The listing builds one solid part. Answer for the finished solid, in the listing's coordinates (mm). A direction names the side the tool comes from. Round coordinates to 2 decimals unless told otherwise and drop trailing zeros. Loops run counter-clockwise (first coordinate to the right, second up) from the corner with the lowest first, then second, coordinate; pieces in that order, holes last. Notation, with made-up numbers: (-3, 28) -> (16, 28) arc R29 ccw to (16, 59) -> close; hole circle Ø11 at (39.5, -14.5). An arc over 180 degrees is marked (long way). Use a Markdown table: item, result. Add a question column.
Q1. Section C-C on z = 8 is taken. Give the vertices of the cut face in (x, y).
Q2. Consider line 1 (X direction, y = 1.5, z = -14); line 2 (X direction, y = 1.25, z = 44); line 3 (X direction, y = 4.25, z = 44). Determine where each line is inside the solid, lowest interval first.
Q3. Section D-D on z = -10.5 is taken. Give the vertices of the cut face in (x, y), then the cut area to 3 significant figures.
Q4. Which of the six approach directions +Z, -Z, +X, -X, +Y, -Y give full straight-line access (tool end or side, diameter ignored) to faces 1 (the flat face through (-34, 9, 25)), 2 (the flat face through (-25.3, 5, -14)), 3 (the flat face through (39, 8, 1)), 4 (the flat face through (42.8, 3, -42.8))?
Q5. Section A-A on x = -44 is taken. Give the vertices of the cut face in (y, z), then the cut area to 3 significant figures.
Q6. Section B-B on z = -44 is taken. Give the vertices of the cut face in (x, y).
Q7. For a pull along X with two mould halves and no side action, classify faces 5 (the flat face through (8, 10, -9)), 6 (the flat face through (-16.4, 5, -14)), 7 (the flat face through (49, 2, 1)) as released by +X, released by -X, zero draft, split by the parting line, or undercut.
Q8. Given pin 1 Ø2 at (y, z) = (9, 27) entering from -X; pin 2 Ø6.5 at (x, z) = (44, 44) entering from +Y; pin 3 Ø1 at (x, z) = (-9, 13.5) entering from +Y, each flat-ended and moving along its own axis, determine where each tip first touches the part or whether it passes through.
from build123d import *

# Parameters (mm, degrees)
SKETCH1_W           = 98
SKETCH1_H           = 98
BOSS_EXTRUDE2_DEPTH = 10
SKETCH2_W           = 98
SKETCH2_H           = 98
SKETCH2_W_2         = 78
SKETCH2_H_2         = 78
CUT_EXTRUDE2_DEPTH  = 5
SKETCH3_R           = 2.75
CUT_EXTRUDE3_DEPTH  = 2
SKETCH4_R           = 1.5
CUT_EXTRUDE4_DEPTH  = 9
SKETCH6_W           = 50
SKETCH6_H           = 28
CUT_EXTRUDE6_DEPTH  = 2.5
CUT_EXTRUDE8_DEPTH  = 11.5


with BuildPart() as part:
    # Sketch1 → Boss-Extrude2 (new body)
    with BuildSketch(Plane(origin=(0, 0, 0), x_dir=(1, 0, 0), z_dir=(0, 1, 0))):
        Rectangle(SKETCH1_W, SKETCH1_H)
    extrude(amount=BOSS_EXTRUDE2_DEPTH)

    # Sketch2 → Cut-Extrude2 (cut)
    with BuildSketch(Plane(origin=(0, 10, 0), x_dir=(1, 0, 0), z_dir=(0, 1, 0))):
        Rectangle(SKETCH2_W, SKETCH2_H)
        Rectangle(SKETCH2_W_2, SKETCH2_H_2, mode=Mode.SUBTRACT)
    extrude(amount=-CUT_EXTRUDE2_DEPTH, mode=Mode.SUBTRACT)

    # Sketch3 → Cut-Extrude3 (cut)
    with BuildSketch(Plane(origin=(0, 5, 0), x_dir=(1, 0, 0), z_dir=(0, 1, 0))):
        with Locations(Location((-44, -44, 0), (0, 0, 270))):
            Circle(SKETCH3_R)
        with Locations(Location((44, -44, 0), (0, 0, 270))):
            Circle(SKETCH3_R)
        with Locations(Location((-44, 44, 0), (0, 0, 270))):
            Circle(SKETCH3_R)
        with Locations(Location((44, 44, 0), (0, 0, 270))):
            Circle(SKETCH3_R)
    extrude(amount=-CUT_EXTRUDE3_DEPTH, mode=Mode.SUBTRACT)

    # Sketch4 → Cut-Extrude4 (cut)
    with BuildSketch(Plane(origin=(0, 3, 0), x_dir=(1, 0, 0), z_dir=(0, 1, 0))):
        with Locations(Location((-44, 44, 0), (0, 0, 270))):
            Circle(SKETCH4_R)
        with Locations(Location((44, 44, 0), (0, 0, 270))):
            Circle(SKETCH4_R)
        with Locations(Location((44, -44, 0), (0, 0, 270))):
            Circle(SKETCH4_R)
        with Locations(Location((-44, -44, 0), (0, 0, 270))):
            Circle(SKETCH4_R)
    extrude(amount=-CUT_EXTRUDE4_DEPTH, mode=Mode.SUBTRACT)

    # Sketch6 → Cut-Extrude6 (cut)
    with BuildSketch(Plane(origin=(0, 10, 0), x_dir=(1, 0, 0), z_dir=(0, 1, 0))):
        with Locations((-9, -25)):
            Rectangle(SKETCH6_W, SKETCH6_H)
    extrude(amount=-CUT_EXTRUDE6_DEPTH, mode=Mode.SUBTRACT)

    # Sketch7 → Cut-Extrude8 (cut)
    with BuildSketch(Plane(origin=(0, 10, 0), x_dir=(1, 0, 0), z_dir=(0, 1, 0))):
        with BuildLine():
            ThreePointArc((-30.3, 32), (-29.714213562, 33.414213562), (-28.3, 34))
            Line((-28.3, 34), (-27.3, 34))
            ThreePointArc((-27.3, 34), (-25.885786438, 33.414213562), (-25.3, 32))
            Line((-25.3, 32), (-25.3, -4))
            ThreePointArc((-25.3, -4), (-25.885786438, -5.414213562), (-27.3, -6))
            Line((-27.3, -6), (-28.3, -6))
            ThreePointArc((-28.3, -6), (-29.714213562, -5.414213562), (-30.3, -4))
            Line((-30.3, -4), (-30.3, 32))
        make_face()
        with BuildLine():
            ThreePointArc((-14.4, -6), (-15.814213562, -5.414213562), (-16.4, -4))
            Line((-16.4, -4), (-16.4, 32))
            ThreePointArc((-16.4, 32), (-15.814213562, 33.414213562), (-14.4, 34))
            Line((-14.4, 34), (-13.4, 34))
            ThreePointArc((-13.4, 34), (-11.985786438, 33.414213562), (-11.4, 32))
            Line((-11.4, 32), (-11.4, -4))
            ThreePointArc((-11.4, -4), (-11.985786438, -5.414213562), (-13.4, -6))
            Line((-13.4, -6), (-14.4, -6))
        make_face()
        with BuildLine():
            ThreePointArc((-0.5, -6), (-1.914213562, -5.414213562), (-2.5, -4))
            Line((-2.5, -4), (-2.5, 32))
            ThreePointArc((-2.5, 32), (-1.914213562, 33.414213562), (-0.5, 34))
            Line((-0.5, 34), (0.5, 34))
            ThreePointArc((0.5, 34), (1.914213562, 33.414213562), (2.5, 32))
            Line((2.5, 32), (2.5, -4))
            ThreePointArc((2.5, -4), (1.914213562, -5.414213562), (0.5, -6))
            Line((0.5, -6), (-0.5, -6))
        make_face()
        with BuildLine():
            ThreePointArc((13.4, -6), (11.985786438, -5.414213562), (11.4, -4))
            Line((11.4, -4), (11.4, 32))
            ThreePointArc((11.4, 32), (11.985786438, 33.414213562), (13.4, 34))
            Line((13.4, 34), (14.4, 34))
            ThreePointArc((14.4, 34), (15.814213562, 33.414213562), (16.4, 32))
            Line((16.4, 32), (16.4, -4))
            ThreePointArc((16.4, -4), (15.814213562, -5.414213562), (14.4, -6))
            Line((14.4, -6), (13.4, -6))
        make_face()
        with BuildLine():
            ThreePointArc((27.3, -34), (25.885786438, -33.414213562), (25.3, -32))
            Line((25.3, -32), (25.3, -6))
            Line((25.3, -6), (25.3, 32))
            ThreePointArc((25.3, 32), (25.885786438, 33.414213562), (27.3, 34))
            Line((27.3, 34), (28.3, 34))
            ThreePointArc((28.3, 34), (29.714213562, 33.414213562), (30.3, 32))
            Line((30.3, 32), (30.3, -6))
            Line((30.3, -6), (30.3, -32))
            ThreePointArc((30.3, -32), (29.714213562, -33.414213562), (28.3, -34))
            Line((28.3, -34), (27.3, -34))
        make_face()
    extrude(amount=-CUT_EXTRUDE8_DEPTH, mode=Mode.SUBTRACT)


solid = part.part
Checked values:
| question | item | result |
|---|---|---|
| 1 | outline | (-49, 0) -> (25.3, 0) -> (25.3, 10) -> (-39, 10) -> (-39, 5) -> (-49, 5) -> close; (30.3, 0) -> (49, 0) -> (49, 5) -> (39, 5) -> (39, 10) -> (30.3, 10) -> close |
| 2 | line 1 | x = -49 to -30.3, -25.3 to -16.4, -11.4 to -2.5, 2.5 to 11.4, 16.4 to 25.3, 30.3 to 49 |
| 2 | line 2 | x = -49 to -45.5, -42.5 to 42.5, 45.5 to 49 |
| 2 | line 3 | x = -49 to -46.75, -41.25 to 41.25, 46.75 to 49 |
| 3 | outline | (-49, 0) -> (-30.3, 0) -> (-30.3, 10) -> (-39, 10) -> (-39, 5) -> (-49, 5) -> close; (-25.3, 0) -> (-16.4, 0) -> (-16.4, 10) -> (-25.3, 10) -> close; (-11.4, 0) -> (-2.5, 0) -> (-2.5, 10) -> (-11.4, 10) -> close; (2.5, 0) -> (11.4, 0) -> (11.4, 10) -> (2.5, 10) -> close; (16.4, 0) -> (25.3, 0) -> (25.3, 10) -> (16.4, 10) -> close; (30.3, 0) -> (49, 0) -> (49, 5) -> (39, 5) -> (39, 10) -> (30.3, 10) -> close |
| 3 | area | 630 mm2 |
| 4 | face 1 | +Z, +Y |
| 4 | face 2 | +Y, -Y |
| 4 | face 3 | +Z, -Z, +X, +Y |
| 4 | face 4 | +Y |
| 5 | outline | (0, -49) -> (5, -49) -> (5, -46.75) -> (3, -46.75) -> (3, -45.5) -> (0, -45.5) -> close; (0, -42.5) -> (3, -42.5) -> (3, -41.25) -> (5, -41.25) -> (5, 41.25) -> (3, 41.25) -> (3, 42.5) -> (0, 42.5) -> close; (0, 45.5) -> (3, 45.5) -> (3, 46.75) -> (5, 46.75) -> (5, 49) -> (0, 49) -> close |
| 5 | area | 450 mm2 |
| 6 | outline | (-49, 0) -> (-45.5, 0) -> (-45.5, 3) -> (-46.75, 3) -> (-46.75, 5) -> (-49, 5) -> close; (-42.5, 0) -> (42.5, 0) -> (42.5, 3) -> (41.25, 3) -> (41.25, 5) -> (-41.25, 5) -> (-41.25, 3) -> (-42.5, 3) -> close; (45.5, 0) -> (49, 0) -> (49, 5) -> (46.75, 5) -> (46.75, 3) -> (45.5, 3) -> close |
| 7 | face 5 | zero draft |
| 7 | face 6 | undercut |
| 7 | face 7 | released by +X |
| 8 | pin 1 | stops at x = -39 |
| 8 | pin 2 | stops at y = 5 |
| 8 | pin 3 | stops at y = 7.5 |
